from build123d import *

# Parameters (mm, degrees)
CUT_EXTRUDE1_DEPTH = 24.500448921
CIRPATTERN1_COUNT  = 12


with BuildPart() as part:
    # Sketch1 → Base-Revolve (revolve)
    with BuildSketch(Plane(origin=(0, 0, 0), x_dir=(0, 0, -1), z_dir=(1, 0, 0))):
        Polygon((8.5, 0), (15.1, 6.6), (15.948528137, 6.6), (9.348528137, 0), align=None)
    revolve(axis=Axis((0, -30, 0), (0, 1, 0)))

    # Sketch2 → Cut-Extrude1 (cut, through all)
    with BuildSketch(Plane.XY):
        Polygon((-0.51, 3.3), (0.51, 3.3), (1.02, 7.6), (-1.02, 7.6), align=None)
    cut_extrude1 = extrude(amount=-CUT_EXTRUDE1_DEPTH, mode=Mode.SUBTRACT)

    # CirPattern1: Cut-Extrude1 ×12 about axis
    cirpattern1_axis = Axis((0, 0, 0), (0, 1, 0))
    for i in range(1, CIRPATTERN1_COUNT):
        add(cut_extrude1.rotate(cirpattern1_axis, i * 360 / CIRPATTERN1_COUNT), mode=Mode.SUBTRACT)


solid = part.part
Can you work these out from the model? Positions are in its coordinate system, mm. A direction names the side the tool comes from. Round coordinates to 2 decimals unless told otherwise and drop trailing zeros. Write each loop counter-clockwise with the first axis right and the second up, starting at its lowest first coordinate (ties: lowest second). Pieces come first, ordered by that corner, then holes. Notation, with made-up numbers: M 32.5,57 L 63.5,57 A23 cw 63.5,67 Z; hole C 84,-14.5 d3. An arc over 180 degrees is marked long. Use a Markdown table: item, result.
Item 1: I want a section at D-D (y = 1.25). List the corners of the cut face in (x, z) for me.
Found:
| item | result |
|---|---|
| outline | C 0,0 d21.2; hole C 0,0 d19.5 |
Item 2: If I drill on line 1 along Z through (x, y) = (9.5, 3.5); line 2 along Z through (x, y) = (-5, 2); line 3 along X through (y, z) = (2.25, -1.5), over which ranges is the centre line in solid material (lowest first)? Write a range as [from, to].
Found:
| item | result |
|---|---|
| line 1 | z = [-8.65, -7.33], [7.33, 8.65] |
| line 2 | z = [-10.19, -9.23], [9.23, 10.19] |
| line 3 | x = [-11.5, -10.64], [10.64, 11.5] |
Item 3: I want a section at A-A (x = 0). List the corners of the cut face in (y, z) for me.
Found:
| item | result |
|---|---|
| outline | M 0,-9.35 L 3.3,-12.65 L 3.3,-11.8 L 0,-8.5 Z; M 0,8.5 L 3.3,11.8 L 3.3,12.65 L 0,9.35 Z |
Item 4: I want a section at C-C (y = 5). State how many separate pieces and enclosed holes the cut face has, and give its area (3 significant figures).
Found:
| item | result |
|---|---|
| separate pieces | 12 |
| enclosed holes | 0 |
| area | 59.7 mm2 |
Item 5: I want a section at B-B (z = 0). List the corners of the cut face in (x, y) for me, and give its area (3 significant figures).
Found:
| item | result |
|---|---|
| outline | M -12.65,3.3 L -9.35,0 L -8.5,0 L -11.8,3.3 Z; M 8.5,0 L 9.35,0 L 12.65,3.3 L 11.8,3.3 Z |
| area | 5.60 mm2 |
Item 6: We'd pull the mould along Z, two halves only. Please class faces 1 (the face through (13.846, 4.958, -0.707)), 2 (the face through (-2.9, 0.3, -9.2)), 3 (the face through (-4, 6.6, -15)), 4 (the face through (-7.535, 4.958, -11.638)): released by +Z, released by -Z, zero draft, split by the parting line, or undercut.
Found:
| item | result |
|---|---|
| face 1 | undercut |
| face 2 | split by the parting line |
| face 3 | zero draft |
| face 4 | released by -Z |
Item 7: For pin 1 Ø2 at (x, z) = (10.5, 12.5) entering from +Y; pin 2 Ø1.5 at (x, y) = (9, 6) entering from +Z; pin 3 Ø0.9 at (x, z) = (12, 0) entering from +Y; pin 4 Ø3 at (x, z) = (-11, -6) entering from -Y, each with a flat end and sliding along its axis, tell me the tip position at first contact or that it passes through.
Found:
| item | result |
|---|---|
| pin 1 | stops at y = 6.6 |
| pin 2 | stops at z = 13.34 |
| pin 3 | stops at y = 3.3 |
| pin 4 | stops at y = 1.68 |
Item 8: Which directions (+Z, -Z, +X, -X, +Y, -Y) give clear straight access to the entire face, cutting with the end or side of a thin tool? Please do faces 5 (the face through (-6.1, 3.3, 10.6)), 6 (the face through (-11.638, 4.958, 7.535)), 7 (the face through (-0.7, 4.9, 13.8)), 8 (the face through (-12, 3.3, 0)).
Found:
| item | result |
|---|---|
| face 5 | +Y |
| face 6 | -X, +Y |
| face 7 | +Z, -Z, +Y |
| face 8 | +X, -X, +Y |
